Input: part model. Units: mm. Frame: model coordinates. Face numbers are marked on the shaded views. A direction names the side the tool comes from. Coordinates: 2 decimals unless noted, no trailing zeros. Order: outer loops, then holes, each group sorted by start corner. A loop starts at its lowest first (then second) coordinate and runs counter-clockwise, first axis right, second up. Notation, with made-up numbers: M -18,83 L -8,83 A25 ccw -8,96 Z; hole C -26,8.5 d1. An arc over 180 degrees is marked long. One line per item, written item: value.
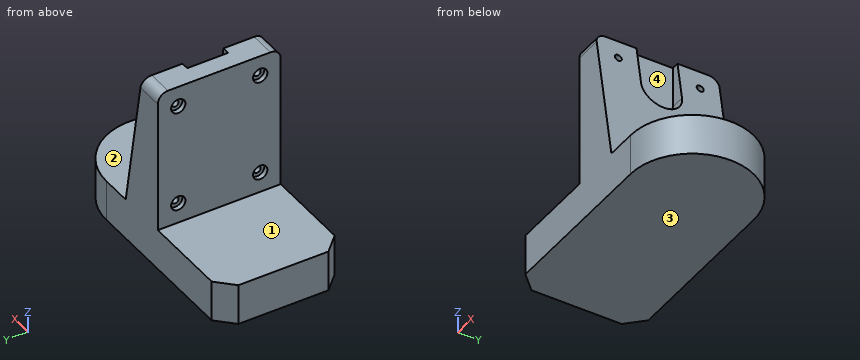
```python
from build123d import *

# Parameters (mm, degrees)
F0_W           = 90
F0_H           = 60
F1_DEPTH       = 20
F2_SIZE        = 8
F4_DEPTH       = 60
F5_R           = 5
F7_D           = 3.4
F7_CBORE_D     = 7
F7_CBORE_DEPTH = 2.4
F9_W           = 20
F9_H           = 20
F10_DEPTH      = 8.9479207717


with BuildPart() as f1:
    # F0 (on Top) → F1 (new body)
    with BuildSketch(Plane.XY):
        with Locations((45, 30)):
            Rectangle(F0_W, F0_H)
        with BuildLine():
            Line((90, 60), (90, 0))
            ThreePointArc((90, 0), (120, 30), (90, 60))
        make_face()
    extrude(amount=F1_DEPTH)

    # F2
    f2_edges = [f1.edges().sort_by_distance(p)[0] for p in [
        (0, 0, 10),
        (0, 60, 10),
    ]]
    chamfer(f2_edges, length=F2_SIZE)

    # F3 (on Front) → F4 (join, through all)
    with BuildSketch(Plane.XZ):
        Polygon((50, 90), (50, 20), (75, 20), (62.6571113504, 90), align=None)
    extrude(amount=-F4_DEPTH)

    # F5
    f5_edges = [f1.edges().sort_by_distance(p)[0] for p in [
        (56.328556, 0, 90),
        (56.328556, 60, 90),
    ]]
    fillet(f5_edges, radius=F5_R)

    # F7 (through all)
    with Locations(Plane(origin=(50, 0, 0), x_dir=(0, -1, 0), z_dir=(-1, 0, 0))):
        with Locations((-50, 80), (-50, 30), (-10, 30), (-10, 80)):
            CounterBoreHole(F7_D / 2, F7_CBORE_D / 2, F7_CBORE_DEPTH)

    # F9 (on offset) → F10 (cut, through all)
    with BuildSketch(Plane(origin=(59, 0, 0), x_dir=(0, -1, 0), z_dir=(-1, 0, 0))):
        with Locations((-30, 80)):
            Rectangle(F9_W, F9_H)
        with BuildLine():
            ThreePointArc((-40, 70), (-30, 60), (-20, 70))
            Line((-20, 70), (-40, 70))
        make_face()
    extrude(amount=-F10_DEPTH, mode=Mode.SUBTRACT)


solid = f1.part
```
(1) Ray query, line 1 (Y direction, x = 61, z = 30); line 2 (Z direction, x = 51.55, y = 10); line 3 (Y direction, x = 62, z = 80). Return the intervals inside material, ascending. Write a range as from..to.
Data:
line 1: y = 0..8.3, 11.7..48.3, 51.7..60
line 2: z = 0..26.5, 33.5..76.5, 83.5..90
line 3: y = 0..8.3, 11.7..20, 40..48.3, 51.7..60
(2) Cut plane B-B on z = 30. Output: boundary loops of the cut face in (x, y).
Data:
outline: M 50,0 L 73.24,0 L 73.24,8.3 L 52.4,8.3 L 52.4,6.5 L 50,6.5 Z; M 50,13.5 L 52.4,13.5 L 52.4,11.7 L 73.24,11.7 L 73.24,48.3 L 52.4,48.3 L 52.4,46.5 L 50,46.5 Z; M 50,53.5 L 52.4,53.5 L 52.4,51.7 L 73.24,51.7 L 73.24,60 L 50,60 Z
(3) Cut plane D-D on x = 71. Output: boundary loops of the cut face in (y, z).
Data:
outline: M 0,0 L 60,0 L 60,42.69 L 0,42.69 Z; hole C 10,30 d3.4; hole C 50,30 d3.4
(4) First-contact query: pin 1 (5.5 mm diameter, centred on y = 9, z = 81, fed in from -X); pin 2 (6.5 mm diameter, centred on y = 10, z = 80, fed in from -X); pin 3 (4.5 mm diameter, centred on y = 10, z = 30, fed in from +X); pin 4 (12 mm diameter, centred on x = 38.5, z = 39, fed in from -Y). Flat tips, straight axial feed; report the tip coordinate or a pass-through.
Data:
pin 1: stops at x = 50
pin 2: stops at x = 52.4
pin 3: stops at x = 73.63
pin 4: passes through
(5) Access query for the marked faces 1, 2, 3 and 4. Directions: +Z, -Z, +X, -X, +Y, -Y. A direction counts if a zero-diameter tool reaches every point of the face in a straight line with its end or side. Return the directions, or none.
Data:
face 1: +Z, -X, +Y, -Y
face 2: +Z, +X, +Y, -Y
face 3: -Z, +X, -X, +Y, -Y
face 4: +Z, +X
(6) Cut plane A-A on y = 50. Output: boundary loops of the cut face in (x, z).
Data:
outline: M 0,0 L 112.36,0 L 112.36,20 L 75,20 L 73.54,28.3 L 52.4,28.3 L 52.4,26.5 L 50,26.5 L 50,20 L 0,20 Z; M 50,33.5 L 52.4,33.5 L 52.4,31.7 L 72.94,31.7 L 64.72,78.3 L 52.4,78.3 L 52.4,76.5 L 50,76.5 Z; M 50,83.5 L 52.4,83.5 L 52.4,81.7 L 64.12,81.7 L 62.66,90 L 50,90 Z
(7) Cut plane C-C on y = 30. Output: boundary loops of the cut face in (x, z).
Data:
outline: M 0,0 L 120,0 L 120,20 L 75,20 L 67.95,60 L 59,60 L 59,90 L 50,90 L 50,20 L 0,20 Z
